from build123d import *

# Parameters (mm, degrees)
BOSS_EXTRUDE2_DEPTH = 38.1
SKETCH1_W           = 25.35
SKETCH1_H           = 28.36
BOSS_EXTRUDE3_DEPTH = 3.81
SKETCH3_W           = 10
SKETCH3_H           = 10
CUT_EXTRUDE1_DEPTH  = 43.860132991
SKETCH4_W           = 7.62
SKETCH4_H           = 30.1
CUT_EXTRUDE2_DEPTH  = 47.084775143
SKETCH5_R           = 1.5
CUT_EXTRUDE3_DEPTH  = 47.084775143
SKETCH6_R           = 1.45
CUT_EXTRUDE4_DEPTH  = 24.344


with BuildPart() as part:
    # Sketch2 → Boss-Extrude2 (new body)
    with BuildSketch(Plane(origin=(0, 0, 0), x_dir=(1, 0, 0), z_dir=(0, 1, 0))):
        Polygon((-9.5, -11.43), (9.5, -11.43), (9.5, -5.08), (12.04, -5.08), (12.04, -13.93), (-13.31, -13.93), (-13.31, 14.43), (12.04, 14.43), (12.04, 7.62), (9.5, 7.62), (9.5, 11.43), (-9.5, 11.43), align=None)
    extrude(amount=BOSS_EXTRUDE2_DEPTH)

    # Sketch1 → Boss-Extrude3 (add)
    with BuildSketch(Plane(origin=(0, 0, 0), x_dir=(1, 0, 0), z_dir=(0, 1, 0))):
        with Locations((-0.635, 0.25)):
            Rectangle(SKETCH1_W, SKETCH1_H)
    extrude(amount=-BOSS_EXTRUDE3_DEPTH)

    # Sketch3 → Cut-Extrude1 (cut, through all)
    with BuildSketch(Plane(origin=(0, 0, 0), x_dir=(1, 0, 0), z_dir=(0, 1, 0))):
        Rectangle(SKETCH3_W, SKETCH3_H)
    extrude(amount=-CUT_EXTRUDE1_DEPTH, mode=Mode.SUBTRACT)

    # Sketch4 → Cut-Extrude2 (cut, through all)
    with BuildSketch(Plane(origin=(-9.5, 0, 0), x_dir=(0, 0, -1), z_dir=(1, 0, 0))):
        with Locations((0, 23.05)):
            Rectangle(SKETCH4_W, SKETCH4_H)
    extrude(amount=-CUT_EXTRUDE2_DEPTH, mode=Mode.SUBTRACT)

    # Sketch5 → Cut-Extrude3 (cut, through all)
    with BuildSketch(Plane(origin=(-9.5, 0, 0), x_dir=(0, 0, -1), z_dir=(1, 0, 0))):
        with Locations((-9.1700096, 31)):
            Circle(SKETCH5_R)
        with Locations((8.3299904, 31)):
            Circle(SKETCH5_R)
    extrude(amount=-CUT_EXTRUDE3_DEPTH, mode=Mode.SUBTRACT)

    # Sketch6 → Cut-Extrude4 (cut)
    with BuildSketch(Plane.XY.offset(13.93)):
        with Locations(Location((-11.405, 19.05, 0), (0, 0, 90))):
            Circle(SKETCH6_R)
        with Locations((-3.81, -1.905)):
            Circle(SKETCH6_R)
    extrude(amount=-CUT_EXTRUDE4_DEPTH, mode=Mode.SUBTRACT)


solid = part.part
For this review, take the finished solid that the model builds, in its own axes (mm). A direction names the side the tool comes from. Coordinates: 2 decimals unless noted, no trailing zeros. Order: outer loops, then holes, each group sorted by start corner. A loop starts at its lowest first (then second) coordinate and runs counter-clockwise, first axis right, second up. Notation, with made-up numbers: (-29, 38) - (-4, 38) arc R11 cw to (-4, 47) - close; hole circle Ø3 at (-17.5, -6). An arc over 180 degrees is marked (long way). Use one line per item in the form item = value.
Q1. Draft analysis for pull direction X (two halves, no side actions). For faces 5 (the flat face through (-9.5, 19, -5)), 6 (the flat face through (-11, 23, 3.81)), state which applies: +X half, -X half, draft (parallel to the pull), parting line (faces both ways), or undercut.
Checked values:
face_5 = undercut
face_6 = draft
Q2. Consider section A-A (y = 19.05). Give the boundary of the cut face in (x, z) (3 decimals).
Checked values:
outline = (-13.31, -14.43) - (12.04, -14.43) - (12.04, -7.62) - (9.5, -7.62) - (9.5, -11.43) - (-9.5, -11.43) - (-9.5, -3.81) - (-9.955, -3.81) - (-9.955, -10.414) - (-12.855, -10.414) - (-12.855, -3.81) - (-13.31, -3.81) - close; (-13.31, 3.81) - (-12.855, 3.81) - (-12.855, 13.93) - (-13.31, 13.93) - close; (-9.955, 3.81) - (-9.5, 3.81) - (-9.5, 11.43) - (9.5, 11.43) - (9.5, 5.08) - (12.04, 5.08) - (12.04, 13.93) - (-9.955, 13.93) - close
Q3. For P1, Ø1, axis at x = 5, z = -6.5, coming from the +Y side; P2, Ø1.7, axis at x = -3.81, y = -1.905, coming from the +Z side; P3, Ø1, axis at y = 9, z = 1, coming from the -X side, all flat-tipped, find the tip position at first contact; note any pin that passes through.
Checked values:
P1 = 0
P2 = -10.41
P3 = through
Q4. For probe 1 along X at (y, z) = (19.05, 8.5) (3 decimals); probe 2 along X at (y, z) = (19.05, -7) (3 decimals); probe 3 along Z at (x, y) = (-7.25, 8), list the stretches that pass through material, from the lowest coordinate up. Write a range as from..to.
Checked values:
probe_1 = -13.31..-12.855, -9.955..-9.5, 9.5..12.04
probe_2 = -13.31..-12.855, -9.955..-9.5
probe_3 = -14.43..-11.43, 11.43..13.93
Q5. For faces 1 (the flat face through (9.5, 19, -9)), 2 (the cylindrical face through (-5.26, -1.84, 1.93)), 3 (the cylindrical face through (-11.378, 30.425, -9.716)), 4 (the flat face through (-11, 23, -3.81)), list the 3-axis set-ups (+Z, -Z, +X, -X, +Y, -Y) from which the entire face can be reached by the end or side of a thin tool; tool diameter is ignored.
Checked values:
face_1 = +Y
face_2 = +Z
face_3 = -X
face_4 = +X, -X, +Y
Q6. Consider section B-B (x = -3.81). Give the boundary of the cut face in (y, z) (3 decimals), then the cut area to 3 significant figures.
Checked values:
outline = (-3.81, -14.43) - (38.1, -14.43) - (38.1, -11.43) - (0, -11.43) - (0, -5) - (-0.455, -5) - (-0.455, -10.414) - (-3.355, -10.414) - (-3.355, -5) - (-3.81, -5) - close; (-3.81, 5) - (-3.355, 5) - (-3.355, 13.93) - (-3.81, 13.93) - close; (-0.455, 5) - (0, 5) - (0, 11.43) - (38.1, 11.43) - (38.1, 13.93) - (-0.455, 13.93) - close
area = 238 mm2
Q7. Consider section D-D (y = 14). Give the boundary of the cut face in (x, z), then the cut area to 3 significant figures.
Checked values:
outline = (-13.31, -14.43) - (12.04, -14.43) - (12.04, -7.62) - (9.5, -7.62) - (9.5, -11.43) - (-9.5, -11.43) - (-9.5, -3.81) - (-13.31, -3.81) - close; (-13.31, 3.81) - (-9.5, 3.81) - (-9.5, 11.43) - (9.5, 11.43) - (9.5, 5.08) - (12.04, 5.08) - (12.04, 13.93) - (-13.31, 13.93) - close
area = 223 mm2
